Here's how the part is built. I have some questions about the finished solid (model axes, mm). A direction names the side the tool comes from. Round coordinates to 2 decimals unless told otherwise and drop trailing zeros. Write each loop counter-clockwise with the first axis right and the second up, starting at its lowest first coordinate (ties: lowest second). Pieces come first, ordered by that corner, then holes. Notation, with made-up numbers: (80, 2.5) -> (124, 2.5) arc R16 ccw to (124, 23.5) -> close; hole circle Ø7 at (-20, 1). An arc over 180 degrees is marked (long way). Answer in a Markdown table with one row per item.
from build123d import *

# Parameters (mm, degrees)
SKETCH1_W           = 5
SKETCH1_H           = 250
BOSS_EXTRUDE1_DEPTH = 10
SKETCH3_R           = 10
BOSS_EXTRUDE2_DEPTH = 10
SKETCH4_R           = 1.5
SKETCH4_R_2         = 1.75
CUT_EXTRUDE1_DEPTH  = 23
EXTRUDE_THIN5_START = -10
EXTRUDE_THIN5_DEPTH = 10
SKETCH10_W          = 5
SKETCH10_H          = 27.5
BOSS_EXTRUDE3_DEPTH = 10
BOSS_EXTRUDE4_DEPTH = 10
SKETCH12_R          = 5.535533906
SKETCH12_R_2        = 3.535533906
EXTRUDE_THIN6_DEPTH = 10
SKETCH14_R          = 3.535533906
CUT_EXTRUDE2_DEPTH  = 10


# Read off the part's stored shape, not the designer's step: Extrude-Thin5
with BuildPart() as part:
    # Sketch1 → Boss-Extrude1 (new body)
    with BuildSketch(Plane(origin=(0, 0, 0), x_dir=(0, 0, -1), z_dir=(1, 0, 0))):
        Rectangle(SKETCH1_W, SKETCH1_H)
    extrude(amount=BOSS_EXTRUDE1_DEPTH)

    # Sketch3 → Boss-Extrude2 (add)
    with BuildSketch(Plane.ZY):
        with Locations((0, -115)):
            Circle(SKETCH3_R)
    extrude(amount=-BOSS_EXTRUDE2_DEPTH)

    # Sketch4 → Cut-Extrude1 (cut)
    with BuildSketch(Plane.ZY):
        with Locations((0, -115)):
            Circle(SKETCH4_R)
        with Locations((-7, -115)):
            Circle(SKETCH4_R_2)
        with Locations((0, -108)):
            Circle(SKETCH4_R_2)
        with Locations((7, -115)):
            Circle(SKETCH4_R_2)
        with Locations((0, -122)):
            Circle(SKETCH4_R_2)
    extrude(amount=-CUT_EXTRUDE1_DEPTH, mode=Mode.SUBTRACT)

    # Extrude-Thin5 outline → Extrude-Thin5 (add)
    with BuildSketch(Plane(origin=(10, 0, 0), x_dir=(0, 0, -1), z_dir=(1, 0, 0)).offset(EXTRUDE_THIN5_START)):
        Polygon((17.451133042, 150.459060521), (2.5, 135.186573848), (2.5, 184.059108288), (-2.5, 184.059108288), (-2.5, 135.005040385), (-17.902207713, 150.083164962), (-21.399952233, 146.51024133), (-2.5, 128.007969476), (-2.5, 125), (2.5, 125), (2.5, 128.039110715), (21.024056673, 146.961316001), align=None)
    extrude(amount=EXTRUDE_THIN5_DEPTH)

    # Sketch10 → Boss-Extrude3 (add)
    with BuildSketch(Plane(origin=(10, 0, 0), x_dir=(0, 0, -1), z_dir=(1, 0, 0))):
        with Locations((18.524056673, 160.711316001)):
            Rectangle(SKETCH10_W, SKETCH10_H)
        Polygon((30.970200678, 156.21277045), (32.755260524, 151.542271403), (18.743763382, 146.187091867), (16.958703537, 150.857590914), align=None)
    extrude(amount=-BOSS_EXTRUDE3_DEPTH)

    # Sketch11 → Boss-Extrude4 (add)
    with BuildSketch(Plane(origin=(10, 0, 0), x_dir=(0, 0, -1), z_dir=(1, 0, 0))):
        Polygon((-21.399952233, 176.51024133), (-21.399952233, 150.083164962), (-17.902207713, 150.083164962), (-16.399952233, 148.612518954), (-16.399952233, 176.51024133), align=None)
        Polygon((-17.902207713, 150.083164962), (-21.399952233, 146.51024133), (-17.902207713, 146.51024133), align=None)
        Polygon((-21.399952233, 150.083164962), (-21.399952233, 146.51024133), (-17.902207713, 150.083164962), align=None)
        Polygon((-17.902207713, 150.083164962), (-17.902207713, 146.51024133), (-16.399952233, 146.51024133), (-16.399952233, 148.612518954), align=None)
        Polygon((-19.942202859, 145.083164962), (-21.399952233, 146.51024133), (-21.399952233, 150.083164962), (-35.402207713, 150.083164962), (-35.402207713, 145.083164962), align=None)
        Polygon((-17.902207713, 146.51024133), (-21.399952233, 146.51024133), (-19.942202859, 145.083164962), (-17.902207713, 145.083164962), align=None)
    extrude(amount=-BOSS_EXTRUDE4_DEPTH)

    # Sketch12 → Extrude-Thin6 (add)
    # profile 1 of 5: a face of its own
    with BuildSketch(Plane(origin=(10, 0, 0), x_dir=(0, 0, -1), z_dir=(1, 0, 0))):
        with Locations((-18.899952233, 179.01024133)):
            Circle(SKETCH12_R)
        with Locations((-18.899952233, 179.01024133)):
            Circle(SKETCH12_R_2, mode=Mode.SUBTRACT)
    # profile 2 of 5: a face of its own
    with BuildSketch(Plane(origin=(10, 0, 0), x_dir=(0, 0, -1), z_dir=(1, 0, 0))):
        with Locations((0, 186.559108288)):
            Circle(SKETCH12_R)
        with Locations((0, 186.559108288)):
            Circle(SKETCH12_R_2, mode=Mode.SUBTRACT)
    # profile 3 of 5: a face of its own
    with BuildSketch(Plane(origin=(10, 0, 0), x_dir=(0, 0, -1), z_dir=(1, 0, 0))):
        with Locations((18.524056673, 176.961316001)):
            Circle(SKETCH12_R)
        with Locations((18.524056673, 176.961316001)):
            Circle(SKETCH12_R_2, mode=Mode.SUBTRACT)
    # profile 4 of 5: a face of its own
    with BuildSketch(Plane(origin=(10, 0, 0), x_dir=(0, 0, -1), z_dir=(1, 0, 0))):
        with Locations((34.197980125, 154.770050849)):
            Circle(SKETCH12_R)
        with Locations((34.197980125, 154.770050849)):
            Circle(SKETCH12_R_2, mode=Mode.SUBTRACT)
    # profile 5 of 5: a face of its own
    with BuildSketch(Plane(origin=(10, 0, 0), x_dir=(0, 0, -1), z_dir=(1, 0, 0))):
        with Locations((-37.902207713, 147.583164962)):
            Circle(SKETCH12_R)
        with Locations((-37.902207713, 147.583164962)):
            Circle(SKETCH12_R_2, mode=Mode.SUBTRACT)
    extrude(amount=-EXTRUDE_THIN6_DEPTH)

    # Sketch14 → Cut-Extrude2 (cut)
    with BuildSketch(Plane(origin=(10, 0, 0), x_dir=(0, 0, -1), z_dir=(1, 0, 0))):
        with Locations((-37.902207713, 147.583164962)):
            Circle(SKETCH14_R)
        with Locations((-18.899952233, 179.01024133)):
            Circle(SKETCH14_R)
        with Locations((0, 186.559108288)):
            Circle(SKETCH14_R)
        with Locations((18.524056673, 176.961316001)):
            Circle(SKETCH14_R)
        with Locations((34.197980125, 154.770050849)):
            Circle(SKETCH14_R)
    extrude(amount=-CUT_EXTRUDE2_DEPTH, mode=Mode.SUBTRACT)


solid = part.part
1) For pin 1 (3 mm diameter, centred on x = 6.5, z = 6.5, fed in from -Y); pin 2 (1 mm diameter, centred on x = 1.5, y = 150, fed in from -Z); pin 3 (5 mm diameter, centred on x = 3, z = 27, fed in from +Y), each with a flat end and sliding along its axis, tell me the tip position at first contact or that it passes through.
Response:
| item | result |
|---|---|
| pin 1 | stops at y = -123.66 |
| pin 2 | stops at z = -37.72 |
| pin 3 | stops at y = 150.08 |
2) We'd pull the mould along Z, two halves only. Please class faces 1 (the face through (5, -115, -10)), 2 (the face through (5, -115, 10)), 3 (the face through (5, 145.083, 27)), 4 (the face through (0, 58, -1)): +Z half, -Z half, draft (parallel to the pull), parting line (faces both ways), or undercut.
Response:
| item | result |
|---|---|
| face 1 | -Z half |
| face 2 | +Z half |
| face 3 | undercut |
| face 4 | draft |
3) I want a section at B-B, the plane x = 5.25. Count the separate pieces of the cut face and the enclosed holes in it, and give its area (3 significant figures).
Response:
| item | result |
|---|---|
| separate pieces | 1 |
| enclosed holes | 10 |
| area | 2,560 mm^2 |
4) I want a section at A-A, the plane y = -35. List the corners of the cut face in (x, z) for me.
Response:
| item | result |
|---|---|
| outline | (0, -2.5) -> (10, -2.5) -> (10, 2.5) -> (0, 2.5) -> close |
5) I need wall thicknesses on line 1 (Y direction, x = 7.25, z = 0); line 2 (Z direction, x = 1, y = 45); line 3 (Y direction, x = 5.5, z = -33). Which ranges of each line are inside material? Lowest first, please. Write a range as [from, to].
Response:
| item | result |
|---|---|
| line 1 | y = [-125, -123.75], [-120.25, -116.5], [-113.5, -109.75], [-106.25, 183.02], [190.09, 192.09] |
| line 2 | z = [-2.5, 2.5] |
| line 3 | y = [149.37, 151.44], [158.1, 160.17] |
6) Which directions (+Z, -Z, +X, -X, +Y, -Y) give clear straight access to the entire face, cutting with the end or side of a thin tool? Please do faces 5 (the face through (4.93, 137.368, -11.632)), 6 (the face through (5, 162, -21.024)), 7 (the face through (5, -125, 0)).
Response:
| item | result |
|---|---|
| face 5 | -Z, +X, -X |
| face 6 | +X, -X |
| face 7 | +Z, -Z, +X, -X, -Y |
